Answer from the drawing. Dimensions are ordinates in mm from the lowest x, y and z of the part. A direction names the side the tool comes from. Give positions to 0.01 mm unless a question says otherwise; leave off trailing zeros. Loops run counter-clockwise (first coordinate to the right, second up) from the corner with the lowest first, then second, coordinate; pieces in that order, holes last.
Item 1: Section A-A, the plane y = 5 is taken. Give the vertices of the cut face in (x, z), and give its area (3 significant figures).
Item 2: A tool of negligible diameter and unlimited length cuts with its end or side. For the marked faces 4 and 5, from which of +Z, -Z, +X, -X, +Y, -Y can it reach the whole face along a straight path? Write none if from no direction.
Item 3: Section D-D, the plane y = 29.7 is taken. Give the vertices of the cut face in (x, z).
Item 4: Consider line 1 along Z through (x, y) = (4, 10.5); line 2 along Z through (x, y) = (0.6, 76.2). Determine where each line is inside the solid, lowest interval first.
Item 5: This flat-tipped pin is pushed along its axis until it touches: pin 1 Ø2.5 at (x, y) = (5, 66.7) entering from +Z. Where does it stop, or does it pass through?
Item 6: The mould has two halves that part along X. Classify the marked faces 1, 2 and 3: pulls with the +X half, pulls with the -X half, needs draft (parallel to the pull), parting line crosses it, or undercut.
Item 7: Section C-C, the plane x = 7.25 is taken. Give the vertices of the cut face in (y, z), and give its area (3 significant figures).
Item 8: Section B-B, the plane z = 1.75 is taken. Give the vertices of the cut face in (x, y), and give its area (3 significant figures).
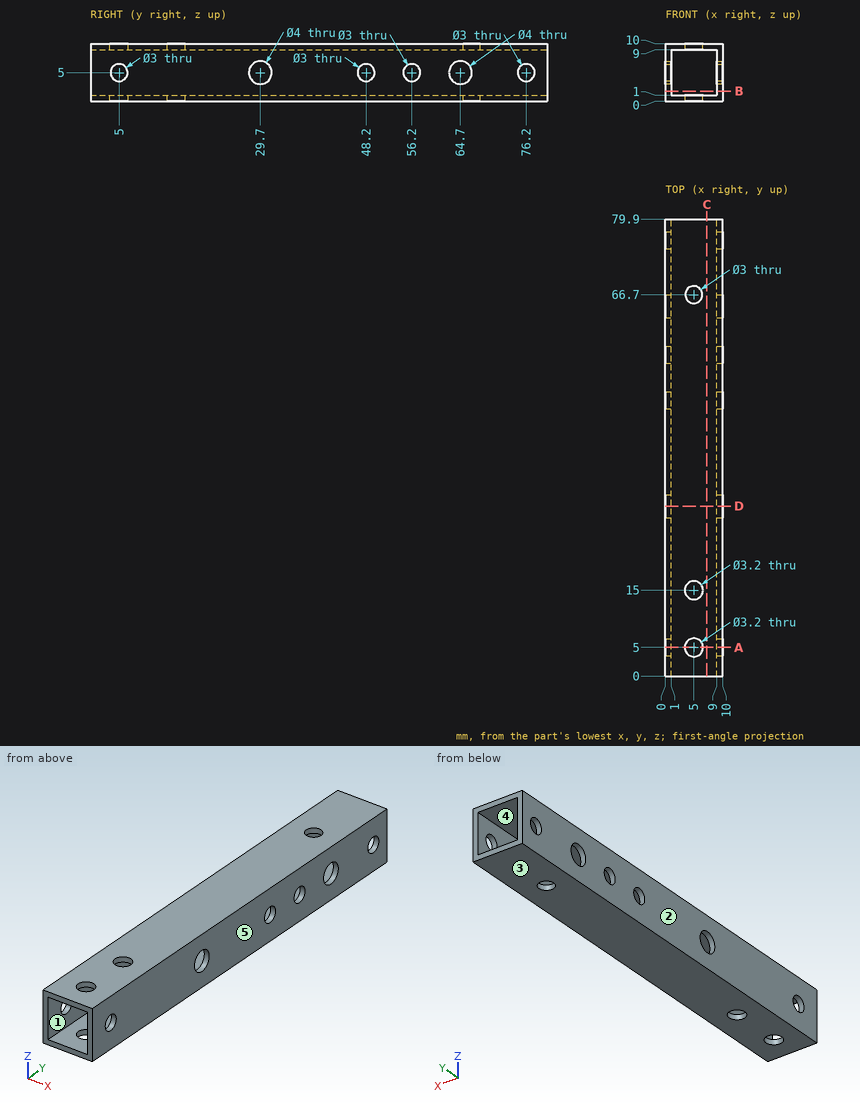
Worked answers:
1. outline: (0, 0) - (3.4, 0) - (3.4, 1) - (1, 1) - (1, 3.5) - (0, 3.5) - close; (0, 6.5) - (1, 6.5) - (1, 9) - (3.4, 9) - (3.4, 10) - (0, 10) - close; (6.6, 0) - (10, 0) - (10, 3.5) - (9, 3.5) - (9, 1) - (6.6, 1) - close; (6.6, 9) - (9, 9) - (9, 6.5) - (10, 6.5) - (10, 10) - (6.6, 10) - close
1. area: 23.6 mm2
2. face 4: +Y, -Y
2. face 5: +Z, -Z, +X, +Y, -Y
3. outline: (0, 0) - (10, 0) - (10, 3) - (9, 3) - (9, 1) - (1, 1) - (1, 3) - (0, 3) - close; (0, 7) - (1, 7) - (1, 9) - (9, 9) - (9, 7) - (10, 7) - (10, 10) - (0, 10) - close
4. line 1: z = 0 to 1, 9 to 10
4. line 2: z = 0 to 3.5, 6.5 to 10
5. pin 1: passes through
6. face 1: undercut
6. face 2: pulls with the -X half
6. face 3: needs draft
7. outline: (0, 0) - (79.9, 0) - (79.9, 1) - (0, 1) - close; (0, 9) - (79.9, 9) - (79.9, 10) - (0, 10) - close
7. area: 160 mm2
8. outline: (0, 0) - (1, 0) - (1, 79.9) - (0, 79.9) - close; (9, 0) - (10, 0) - (10, 79.9) - (9, 79.9) - close
8. area: 160 mm2
